Part print with two shaded views. Sizes in mm from the minimum x, y, z corner. Give positions to 0.01 mm unless a question says otherwise; leave off trailing zeros. Write each loop counter-clockwise with the first axis right and the second up, starting at its lowest first coordinate (ties: lowest second). Pieces come first, ordered by that corner, then holes. Notation, with made-up numbers: (-21.75, -21.5) - (-1.75, -21.5) arc R32 ccw to (-1.75, 11.5) - close; hole circle Ø1 at (14.5, -9). An arc over 180 degrees is marked (long way). Answer as a JSON object with one key per item and string values.
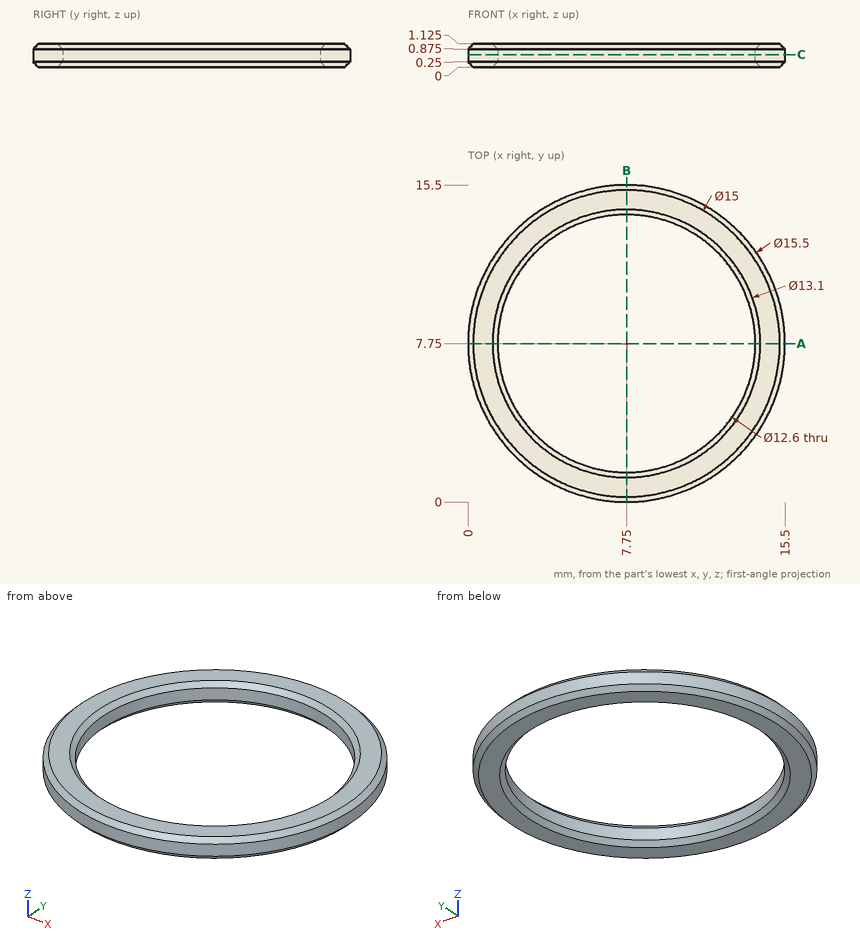
(1) Probe L1, parallel to Y at x = 7.75, z = 0.65; L2, parallel to X at y = 2.5, z = 0.1; L3, parallel to X at y = 9.5, z = 0.1. List the from-to ranges inside material, lowest first. Write a range as [from, to].
Answer key:
{"L1": "y = [0, 1.45], [14.05, 15.5]", "L2": "x = [2.25, 4], [11.5, 13.25]", "L3": "x = [0.35, 1.54], [13.96, 15.15]"}
(2) Saw through at C-C, the plane z = 0.6. Give the cut face in (x, y).
Answer key:
{"outline": "circle Ø15.5 at (7.75, 7.75); hole circle Ø12.6 at (7.75, 7.75)"}
(3) Flat gauge pins, fed straight in: P1, Ø8, axis at x = 10.5, y = 13, coming from the +Z side (3 decimals); P2, Ø5, axis at x = 10, y = 8, coming from the -Z side. Where does each tip first touch, or does it go through?
Answer key:
{"P1": "stops at z = 1.125", "P2": "passes through"}
(4) Saw through at A-A, the plane y = 7.75. Give the cut face in (x, z) (3 decimals), and give its area (3 significant figures).
Answer key:
{"outline": "(0, 0.25) - (0.25, 0) - (1.2, 0) - (1.45, 0.25) - (1.45, 0.875) - (1.2, 1.125) - (0.25, 1.125) - (0, 0.875) - close; (14.05, 0.25) - (14.3, 0) - (15.25, 0) - (15.5, 0.25) - (15.5, 0.875) - (15.25, 1.125) - (14.3, 1.125) - (14.05, 0.875) - close", "area": "3.01 mm²"}
